Input: part model. Units: mm. Frame: model coordinates. A direction names the side the tool comes from. Round coordinates to 2 decimals unless told otherwise and drop trailing zeros. Order: outer loops, then holes, each group sorted by start corner. A loop starts at its lowest first (then second) coordinate and runs counter-clockwise, first axis right, second up.
Item 1: Line query: L1, parallel to X at y = 3.5, z = 0; L2, parallel to X at y = 9, z = -16; L3, parallel to X at y = 12.5, z = -10.5. Output: solid intervals per line, ascending.
Item 2: First-contact query: pin 1 (1.4 mm diameter, centred on y = 6.5, z = -13.5, fed in from +X); pin 2 (2.5 mm diameter, centred on y = 7, z = -14.5, fed in from -X); pin 3 (9.5 mm diameter, centred on y = 6.5, z = -12.5, fed in from +X); pin 4 (5.5 mm diameter, centred on x = 6, z = -16, fed in from +Y). Flat tips, straight axial feed; report the tip coordinate or a pass-through.
Item 3: Reachability of faces 1 (the cylindrical face through (-6.8, 4.2, -16.8)), 2 (the flat face through (-16.22, 4.35, -12.8)), 3 (the flat face through (16.23, 5.92, 11.36)), 4 (the cylindrical face through (7.361, 15.328, -15.323)), 5 (the cylindrical face through (0.782, 15.328, 16.982)) from +Z, -Z, +X, -X, +Y, -Y: full face, straight path, thin tool, end or side. Return the list, or none.
Item 4: Cut plane A-A on z = 0. Output: boundary loops of the cut face in (x, y).
Item 5: Cut plane B-B on x = -22.5. Output: boundary loops of the cut face in (y, z), then the cut area to 3 significant figures.
Item 6: Cut plane C-C on y = 13.75. Output: boundary loops of the cut face in (x, z), then the cut area to 3 significant figures.
Item 7: Mould query, pull axis Z, two halves, no side actions, for faces 6 (the flat face through (-18.009, 7.638, -6.813)), 7 (the flat face through (-16.22, 5.44, -16.63)), 8 (the flat face through (12.8, 6, -14)), 9 (the cylindrical face through (-7.2, 15.3, -15.4)). Classes: released by +Z, released by -Z, zero draft, split by the parting line, or undercut.
Item 8: Cut plane D-D on x = -3. Give the number of separate pieces and of enclosed holes in the cut face, then the cut area to 3 significant figures.
```python
from build123d import *

# Parameters (mm, degrees)
SKETCH1_R                   = 3.4
BOSS_EXTRUDE1_DEPTH         = 12
SKETCH3_R                   = 17
BOSS_EXTRUDE2_DEPTH         = 8
FILLET1_R                   = 1.25
CUT_EXTRUDE1_DEPTH          = 37.78056552
CUT_EXTRUDE1_DEPTH_BACK     = 37.78056552
CUT_EXTRUDE2_DEPTH          = 41.109973918
CUT_EXTRUDE2_DEPTH_BACK     = 41.109973918
SKETCH4_R                   = 10
CUT_EXTRUDE3_DEPTH          = 41.109973918
CUT_EXTRUDE3_DEPTH_BACK     = 41.109973918
SKETCH5_W                   = 2
SKETCH5_H                   = 20
SKETCH7_R                   = 3
CUT_EXTRUDE4_DEPTH          = 12.5
FILLET2_R                   = 3
FILLET3_R                   = 1
M5_TAPPED_HOLE2_D           = 4.2
M5_TAPPED_HOLE2_CSINK_D     = 5.05
M5_TAPPED_HOLE2_CSINK_ANGLE = 90
BOSS_EXTRUDE4_DEPTH         = 0.001
BOSS_EXTRUDE4_DEPTH_BACK    = 25.5
SKETCH26_R                  = 2.5
SKETCH28_R                  = 4
BOSS_EXTRUDE5_DEPTH         = 5
CHAMFER1_SIZE               = 0.125
CUT_EXTRUDE5_DEPTH          = 3
FILLET4_R                   = 0.75


with BuildPart() as part:
    # Sketch1 → Boss-Extrude1 (new body)
    with BuildSketch(Plane(origin=(0, 0, 0), x_dir=(1, 0, 0), z_dir=(0, 1, 0))):
        with BuildLine():
            Line((5, -18.4), (-5, -18.4))
            Line((-5, -18.4), (-26.920975839, -4.66024679))
            ThreePointArc((-26.920975839, -4.66024679), (-29.473599119, -0.538249647), (-27.772784233, 4.002011885))
            Line((-27.772784233, 4.002011885), (-12.5, 18.4))
            Line((-12.5, 18.4), (12.5, 18.4))
            Line((12.5, 18.4), (27.772784233, 4.002011885))
            ThreePointArc((27.772784233, 4.002011885), (29.473599119, -0.538249647), (26.920975839, -4.66024679))
            Line((26.920975839, -4.66024679), (5, -18.4))
        make_face()
        with Locations(Location((-24, 0, 0), (0, 0, 270))):
            Circle(SKETCH1_R, mode=Mode.SUBTRACT)
        with Locations(Location((24, 0, 0), (0, 0, 90))):
            Circle(SKETCH1_R, mode=Mode.SUBTRACT)
    extrude(amount=BOSS_EXTRUDE1_DEPTH)

    # Sketch3 → Boss-Extrude2 (add)
    with BuildSketch(Plane(origin=(0, 12, 0), x_dir=(1, 0, 0), z_dir=(0, 1, 0))):
        with Locations(Location((0, 0, 0), (0, 0, 270))):
            Circle(SKETCH3_R)
    extrude(amount=BOSS_EXTRUDE2_DEPTH)

    # Fillet1
    fillet1_edges = [part.edges().sort_by_distance(p)[0] for p in [
        (0, 20, -17),
    ]]
    fillet(fillet1_edges, radius=FILLET1_R)

    # Sketch2 → Cut-Extrude1 (cut, two sides: drawn at the far end of the back side and taken through both)
    with BuildSketch(Plane(origin=(0, 12, 0), x_dir=(1, 0, 0), z_dir=(0, 1, 0)).offset(-CUT_EXTRUDE1_DEPTH_BACK)):
        Polygon((12.5, 18.4), (12.5, 10.4), (27.772784233, 4.002011885), align=None)
        Polygon((-12.5, 18.4), (-12.5, 8.399645995), (-27.772784233, 4.002011885), align=None)
    extrude(amount=CUT_EXTRUDE1_DEPTH + CUT_EXTRUDE1_DEPTH_BACK, mode=Mode.SUBTRACT)

    # Sketch4 → Cut-Extrude2 (cut, two sides: drawn at the far end of the back side and taken through both)
    with BuildSketch(Plane(origin=(0, 20, 0), x_dir=(1, 0, 0), z_dir=(0, 1, 0)).offset(-CUT_EXTRUDE2_DEPTH_BACK)):
        with Locations(Location((0, 0, 0), (0, 0, 270))):
            Circle(SKETCH4_R)
    extrude(amount=CUT_EXTRUDE2_DEPTH + CUT_EXTRUDE2_DEPTH_BACK, mode=Mode.SUBTRACT)

    # Sketch5 → Cut-Extrude3 (cut, two sides: drawn at the far end of the back side and taken through both)
    with BuildSketch(Plane(origin=(0, 20, 0), x_dir=(1, 0, 0), z_dir=(0, 1, 0)).offset(-CUT_EXTRUDE3_DEPTH_BACK)):
        with Locations((0, 10)):
            Rectangle(SKETCH5_W, SKETCH5_H)
    extrude(amount=CUT_EXTRUDE3_DEPTH + CUT_EXTRUDE3_DEPTH_BACK, mode=Mode.SUBTRACT)

    # Sketch7 → Cut-Extrude4 (cut)
    with BuildSketch(Plane.ZY.offset(12.5)):
        with Locations((-14.4, 6)):
            Circle(SKETCH7_R)
    extrude(amount=-CUT_EXTRUDE4_DEPTH, mode=Mode.SUBTRACT)

    # Fillet2
    fillet2_edges = [part.edges().sort_by_distance(p)[0] for p in [
        (27.772784233, 6, -4.002011885),
        (-27.772784233, 6, -4.002011885),
    ]]
    fillet(fillet2_edges, radius=FILLET2_R)

    # Fillet3
    fillet3_edges = [part.edges().sort_by_distance(p)[0] for p in [
        (5, 6, 18.4),
        (-5, 6, 18.4),
    ]]
    fillet(fillet3_edges, radius=FILLET3_R)

    # M5 Tapped Hole2 (through all)
    with Locations(Plane(origin=(12.5, 0, 0), x_dir=(0, 0, -1), z_dir=(1, 0, 0))):
        with Locations((14.4, 6)):
            CounterSinkHole(M5_TAPPED_HOLE2_D / 2, M5_TAPPED_HOLE2_CSINK_D / 2, counter_sink_angle=M5_TAPPED_HOLE2_CSINK_ANGLE)



with BuildPart() as body_2:
    # Sketch26 → Boss-Extrude4 (new, two sides: drawn at the far end of the back side and taken through both)
    with BuildSketch(Plane.ZY.offset(12.7).offset(-BOSS_EXTRUDE4_DEPTH_BACK)):
        with Locations((-14.4, 6)):
            Circle(SKETCH26_R)
    extrude(amount=BOSS_EXTRUDE4_DEPTH + BOSS_EXTRUDE4_DEPTH_BACK)


with BuildPart() as part_1:
    add(part.part)

    add(body_2.part)  # Boss-Extrude5 merges body 2
    # Sketch28 → Boss-Extrude5 (add)
    with BuildSketch(Plane.ZY.offset(12.701)):
        with Locations((-14.4, 6)):
            Circle(SKETCH28_R)
    extrude(amount=BOSS_EXTRUDE5_DEPTH)

    # Chamfer1
    chamfer1_edges = [part_1.edges().sort_by_distance(p)[0] for p in [
        (12.8, 6, -16.9),
    ]]
    chamfer(chamfer1_edges, length=CHAMFER1_SIZE)

    # Sketch29 → Cut-Extrude5 (cut)
    with BuildSketch(Plane.ZY.offset(17.701)):
        Polygon((-15.067828808, 8.570474279), (-16.960010429, 6.706880427), (-16.292181621, 4.136406148), (-13.732171192, 3.429525721), (-11.839989571, 5.293119573), (-12.507818379, 7.863593852), align=None)
    extrude(amount=-CUT_EXTRUDE5_DEPTH, mode=Mode.SUBTRACT)

    # Fillet4
    fillet4_edges = [part_1.edges().sort_by_distance(p)[0] for p in [
        (-17.701, 6, -18.4),
    ]]
    fillet(fillet4_edges, radius=FILLET4_R)


solid = part_1.part
```
From the geometry:
1. L1: x = -29.5 to -27.4, -20.6 to -10, 10 to 20.6, 27.4 to 29.5
1. L2: x = -17.69 to -12.7, -12.5 to -1, 1 to 12.5
1. L3: x = -12.5 to -1, 1 to 12.5
2. pin 1: stops at x = 12.8
2. pin 2: stops at x = -14.7
2. pin 3: stops at x = 18.83
2. pin 4: stops at y = 20
3. face 1: none
3. face 2: -X
3. face 3: +Z, +X, +Y, -Y
3. face 4: -Z, +X, +Y
3. face 5: +Y
4. outline: (-29.5, 0) - (-27.4, 0) - (-27.4, 12) - (-29.5, 12) - close; (-20.6, 0) - (-10, 0) - (-10, 20) - (-15.75, 20) arc R1.25 ccw to (-17, 18.75) - (-17, 12) - (-20.6, 12) - close; (10, 0) - (20.6, 0) - (20.6, 12) - (17, 12) - (17, 18.75) arc R1.25 ccw to (15.75, 20) - (10, 20) - close; (27.4, 0) - (29.5, 0) - (29.5, 12) - (27.4, 12) - close
5. outline: (0, -5.52) - (12, -5.52) - (12, -3.05) - (0, -3.05) - close; (0, 3.05) - (12, 3.05) - (12, 7.43) - (0, 7.43) - close
5. area: 82.2 mm2
6. outline: (-15.19, -7.62) - (-12.5, -8.4) - (-12.5, -11.52) arc R17 ccw to (-1, -16.97) - (-1, -9.95) arc R10 cw (long way) to (1, -9.95) - (1, -16.97) arc R17 ccw to (12.5, -11.52) - (12.5, -10.4) - (13.87, -9.82) arc R17 ccw (long way) to start
6. area: 574 mm2
7. face 6: undercut
7. face 7: undercut
7. face 8: zero draft
7. face 9: released by -Z
8. separate pieces: 3
8. enclosed holes: 1
8. area: 318 mm2
